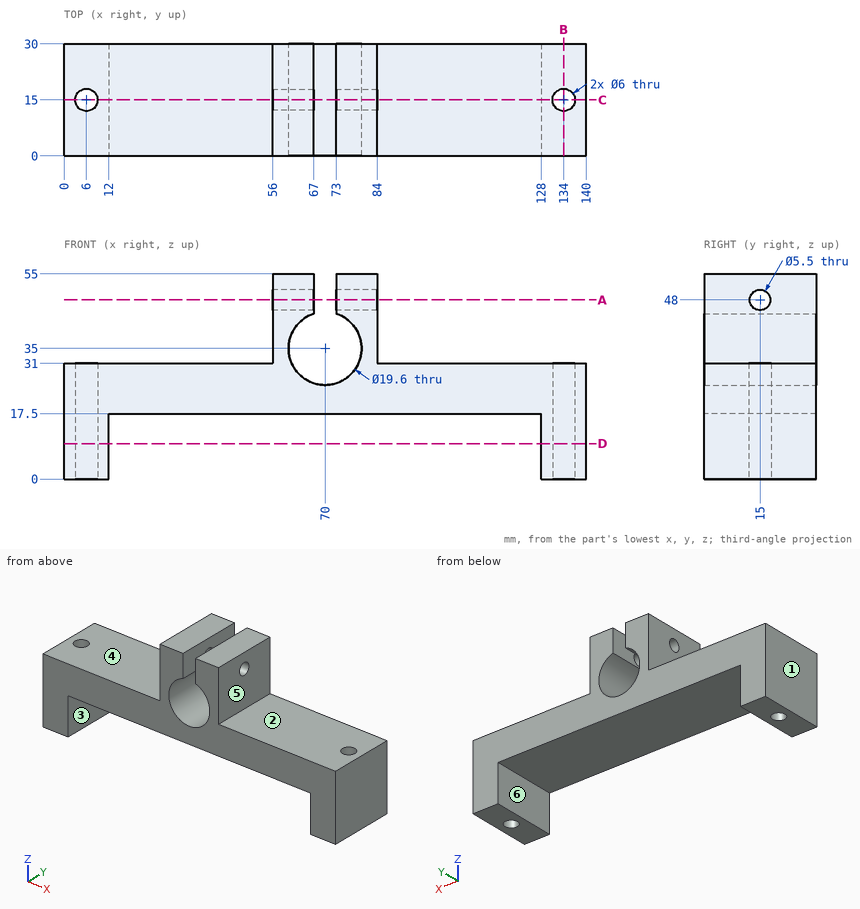
Geometry: see drawing. Coordinates: mm, zero at the bounding-box minimum. A direction names the side the tool comes from. Round coordinates to 2 decimals unless told otherwise and drop trailing zeros. Loops run counter-clockwise (first coordinate to the right, second up) from the corner with the lowest first, then second, coordinate; pieces in that order, holes last.
(1) Material intervals for probe 1 along X at (y, z) = (19.25, 50.5); probe 2 along Y at (x, z) = (134, 18); probe 3 along Z at (x, y) = (51.5, 5), sorted ascending.
From the geometry:
probe 1: x = 56 to 67, 73 to 84
probe 2: y = 0 to 12, 18 to 30
probe 3: z = 17.5 to 31
(2) Section query B-B (x = 134). Output: boundary loops of the cut face in (y, z).
From the geometry:
outline: (0, 0) - (12, 0) - (12, 31) - (0, 31) - close; (18, 0) - (30, 0) - (30, 31) - (18, 31) - close
(3) Section query A-A (z = 48). Output: boundary loops of the cut face in (x, y), and give its area (3 significant figures).
From the geometry:
outline: (56, 0) - (67, 0) - (67, 12.25) - (56, 12.25) - close; (56, 17.75) - (67, 17.75) - (67, 30) - (56, 30) - close; (73, 0) - (84, 0) - (84, 12.25) - (73, 12.25) - close; (73, 17.75) - (84, 17.75) - (84, 30) - (73, 30) - close
area: 539 mm2
(4) Section query C-C (y = 15). Give the number of separate pieces and of enclosed holes in the cut face, and give its area (3 significant figures).
From the geometry:
separate pieces: 5
enclosed holes: 0
area: 2,130 mm2
(5) Pull-direction query (X, two-part tool) for the marked faces 1, 2 and 3; classes: +X half, -X half, draft (parallel to the pull), parting line (faces both ways), or undercut.
From the geometry:
face 1: -X half
face 2: draft
face 3: undercut
(6) Access query for the marked faces 4, 5 and 6. Directions: +Z, -Z, +X, -X, +Y, -Y. A direction counts if a zero-diameter tool reaches every point of the face in a straight line with its end or side. Return the directions, or none.
From the geometry:
face 4: +Z, -X, +Y, -Y
face 5: +Z, +X, +Y, -Y
face 6: -Z, +Y, -Y
(7) Contact query for flat-ended pins moving along their axis: pin 1 Ø5 at (y, z) = (15, 38) entering from +X; pin 2 Ø11.5 at (y, z) = (8, 47) entering from -X; pin 3 Ø15 at (x, y) = (97.5, 8) entering from -Z. Output: stop coordinate, or through.
From the geometry:
pin 1: stops at x = 84
pin 2: stops at x = 56
pin 3: stops at z = 17.5
(8) Section query D-D (z = 9.5). Output: boundary loops of the cut face in (x, y), and give its area (3 significant figures).
From the geometry:
outline: (0, 0) - (12, 0) - (12, 30) - (0, 30) - close; (128, 0) - (140, 0) - (140, 30) - (128, 30) - close; hole circle Ø6 at (6, 15); hole circle Ø6 at (134, 15)
area: 663 mm2
